Read the model definition and answer for the solid it produces. Units are mm, in the model's axes. A direction names the side the tool comes from. Give positions to 0.01 mm unless a question says otherwise; leave off trailing zeros. Order: outer loops, then holes, each group sorted by start corner. A loop starts at its lowest first (then second) coordinate and runs counter-clockwise, first axis right, second up. Notation, with made-up numbers: (-13.75, 86) - (10.25, 86) arc R17 cw to (10.25, 102) - close; hole circle Ø1 at (69, 52.25). An arc over 180 degrees is marked (long way). Use a Markdown table: item, result. Add a question column.
1. Consider L1, parallel to Y at x = 0, z = -1.25; L2, parallel to Y at x = -3.5, z = 14.5; L3, parallel to Y at x = -16.5, z = 1. Determine where each line is inside the solid, lowest interval first.
2. Flat-ended cylindrical pins translate along their axes: P1, Ø8, axis at x = 4.5, y = 17.5, coming from the -Z side; P2, Ø1, axis at x = 10.5, z = 7, coming from the -Y side; P3, Ø2, axis at x = -13.5, y = 17, coming from the +Z side. Find the tip coordinate at first contact, or state that the pin passes through.
3. A cutting plane is placed at B-B on z = 0. Determine the outline of the cut face in (x, y).
4. Which of the six approach directions +Z, -Z, +X, -X, +Y, -Y give full straight-line access (tool end or side, diameter ignored) to faces 4 (the cylindrical face through (-1.8, -22.3, -2.4)), 5 (the flat face through (0, 46, 0)), 6 (the flat face through (15, 23, -6))?
5. A cutting plane is placed at D-D on y = -32. Determine the outline of the cut face in (x, z), and give its area (3 significant figures).
6. A cutting plane is placed at A-A on x = 0. Determine the outline of the cut face in (y, z), and give its area (4 significant figures).
7. For a pull along Y with two mould halves and no side action, classify faces 1 (the flat face through (0, 0, 8)), 2 (the cylindrical face through (-15.62, 34.34, -3.47)), 3 (the cylindrical face through (-1.43, -22.45, -0.04)) as released by +Y, released by -Y, zero draft, split by the parting line, or undercut.
8. A cutting plane is placed at C-C on z = 13.5. Determine the outline of the cut face in (x, y).
```python
from build123d import *

# Parameters (mm, degrees)
SKETCH2_R               = 18.5
BOSS_EXTRUDE1_DEPTH     = 23
SKETCH3_R               = 16
BOSS_EXTRUDE2_DEPTH     = 23
SKETCH4_R               = 7
BOSS_EXTRUDE3_DEPTH     = 8
SKETCH12_R              = 3
BOSS_EXTRUDE6_DEPTH     = 37
CUT_EXTRUDE1_DEPTH      = 10
CUT_EXTRUDE1_DEPTH_BACK = 10
SKETCH7_R               = 1.5


with BuildPart() as part:
    # Sketch2 → Boss-Extrude1 (new body)
    with BuildSketch(Plane(origin=(0, 0, 0), x_dir=(1, 0, 0), z_dir=(0, 1, 0))):
        with Locations(Location((0, 0, 0), (0, 0, 270))):
            Circle(SKETCH2_R)
    extrude(amount=BOSS_EXTRUDE1_DEPTH)

    # Sketch3 → Boss-Extrude2 (add)
    with BuildSketch(Plane(origin=(0, 23, 0), x_dir=(1, 0, 0), z_dir=(0, 1, 0))):
        with Locations(Location((0, 0, 0), (0, 0, 270))):
            Circle(SKETCH3_R)
    extrude(amount=BOSS_EXTRUDE2_DEPTH)

    # Sketch4 → Boss-Extrude3 (add)
    with BuildSketch(Plane.XZ):
        with Locations(Location((0, 0, 0), (0, 0, 270))):
            Circle(SKETCH4_R)
    extrude(amount=BOSS_EXTRUDE3_DEPTH)

    # Sketch12 → Boss-Extrude6 (add)
    with BuildSketch(Plane(origin=(0, 0, 0), x_dir=(1, 0, 0), z_dir=(0, 1, 0))):
        with Locations(Location((0, 0, 0), (0, 0, 270))):
            Circle(SKETCH12_R)
    extrude(amount=-BOSS_EXTRUDE6_DEPTH)

    # Sketch7 → Cut-Extrude1 (cut, two sides: drawn at the far end of the back side and taken through both)
    with BuildSketch(Plane.XY.offset(-CUT_EXTRUDE1_DEPTH_BACK)):
        with Locations(Location((0, -22, 0), (0, 0, 180))):
            Circle(SKETCH7_R)
    extrude(amount=CUT_EXTRUDE1_DEPTH + CUT_EXTRUDE1_DEPTH_BACK, mode=Mode.SUBTRACT)


solid = part.part
```
Output values:
| question | item | result |
|---|---|---|
| 1 | L1 | -37 to -23.5, -20.5 to 46 |
| 1 | L2 | 0 to 46 |
| 1 | L3 | 0 to 23 |
| 2 | P1 | z = -18.49 |
| 2 | P2 | y = 0 |
| 2 | P3 | z = 13.64 |
| 3 | outline | (-18.5, 0) - (-7, 0) - (-7, -8) - (-3, -8) - (-3, -37) - (3, -37) - (3, -8) - (7, -8) - (7, 0) - (18.5, 0) - (18.5, 23) - (16, 23) - (16, 46) - (-16, 46) - (-16, 23) - (-18.5, 23) - close; hole circle Ø3 at (0, -22) |
| 4 | face 4 | -Y |
| 4 | face 5 | +Z, -Z, +X, -X, +Y |
| 4 | face 6 | +Y |
| 5 | outline | circle Ø6 at (0, 0) |
| 5 | area | 28.3 mm² |
| 6 | outline | (-37, -3) - (-23.5, -3) - (-23.5, 3) - (-37, 3) - close; (-20.5, -3) - (-8, -3) - (-8, -7) - (0, -7) - (0, -18.5) - (23, -18.5) - (23, -16) - (46, -16) - (46, 16) - (23, 16) - (23, 18.5) - (0, 18.5) - (0, 7) - (-8, 7) - (-8, 3) - (-20.5, 3) - close |
| 6 | area | 1,855 mm² |
| 7 | face 1 | released by -Y |
| 7 | face 2 | zero draft |
| 7 | face 3 | undercut |
| 8 | outline | (-12.65, 0) - (12.65, 0) - (12.65, 23) - (8.59, 23) - (8.59, 46) - (-8.59, 46) - (-8.59, 23) - (-12.65, 23) - close |
